from build123d import *

# Parameters (mm, degrees)
SKETCH1_R           = 1.5
SKETCH1_R_2         = 1.25
BOSS_EXTRUDE1_DEPTH = 3
SKETCH2_R           = 1.25
BOSS_EXTRUDE2_DEPTH = 3
SKETCH3_R           = 5
SKETCH3_R_2         = 3
BOSS_EXTRUDE3_DEPTH = 5
SKETCH3_2_R         = 3
SKETCH3_2_R_2       = 1.5
BOSS_EXTRUDE4_DEPTH = 1
CHAMFER1_SIZE       = 1.5


with BuildPart() as part:
    # Sketch1 → Boss-Extrude1 (new body)
    with BuildSketch(Plane(origin=(0, 0, 0), x_dir=(1, 0, 0), z_dir=(0, 1, 0))):
        with BuildLine():
            Line((-8.5, 6), (8.5, 6))
            ThreePointArc((8.5, 6), (14.5, 0), (8.5, -6))
            Line((8.5, -6), (-8.5, -6))
            ThreePointArc((-8.5, -6), (-14.5, 0), (-8.5, 6))
        make_face()
        with Locations((-8.5, 0)):
            Circle(SKETCH1_R, mode=Mode.SUBTRACT)
        with Locations((11.25, 0)):
            Circle(SKETCH1_R_2, mode=Mode.SUBTRACT)
        with Locations((6.25, 0)):
            Circle(SKETCH1_R_2, mode=Mode.SUBTRACT)
    extrude(amount=BOSS_EXTRUDE1_DEPTH)

    # Sketch2 → Boss-Extrude2 (add)
    with BuildSketch(Plane(origin=(0, 3, 0), x_dir=(1, 0, 0), z_dir=(0, 1, 0))):
        with BuildLine():
            Line((6, 3), (11.5, 3))
            ThreePointArc((11.5, 3), (14.5, 0), (11.5, -3))
            Line((11.5, -3), (6, -3))
            ThreePointArc((6, -3), (3, 0), (6, 3))
        make_face()
        with Locations((6.25, 0)):
            Circle(SKETCH2_R, mode=Mode.SUBTRACT)
        with Locations((11.25, 0)):
            Circle(SKETCH2_R, mode=Mode.SUBTRACT)
    extrude(amount=BOSS_EXTRUDE2_DEPTH)

    # Sketch3 → Boss-Extrude3 (add)
    with BuildSketch(Plane.XZ):
        with Locations((-8.5, 0)):
            Circle(SKETCH3_R)
        with Locations((-8.5, 0)):
            Circle(SKETCH3_R_2, mode=Mode.SUBTRACT)
    extrude(amount=BOSS_EXTRUDE3_DEPTH)

    # Sketch3<2> → Boss-Extrude4 (add)
    with BuildSketch(Plane.XZ):
        with Locations((-8.5, 0)):
            Circle(SKETCH3_2_R)
        with Locations((-8.5, 0)):
            Circle(SKETCH3_2_R_2, mode=Mode.SUBTRACT)
    extrude(amount=BOSS_EXTRUDE4_DEPTH)

    # Chamfer1
    chamfer1_edges = [part.edges().sort_by_distance(p)[0] for p in [
        (-10, 3, 0),
    ]]
    chamfer(chamfer1_edges, length=CHAMFER1_SIZE)


solid = part.part
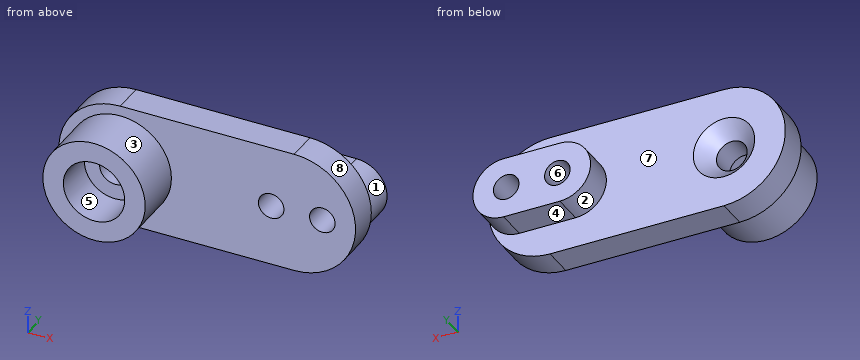
Work out the finished part from the listing and answer in its coordinate system (mm). Face numbers are marked on the shaded views. A direction names the side the tool comes from. Round coordinates to 2 decimals unless told otherwise and drop trailing zeros. Loops run counter-clockwise (first coordinate to the right, second up) from the corner with the lowest first, then second, coordinate; pieces in that order, holes last. Notation, with made-up numbers: (66, 9.5) - (113, 9.5) arc R14 ccw to (113, 31.5) - close; hole circle Ø2 at (23, -17.5). An arc over 180 degrees is marked (long way). Use one line per item in the form item = value. Start each with the question number.
(1) Determine the mould class of the marked faces 5, 6, 7 and 8 for opening direction X: +X half, -X half, draft (parallel to the pull), parting line (faces both ways), or undercut.
(2) Flat-ended cylindrical pins translate along their axes: P1, Ø2, axis at x = -4, z = 3, coming from the +Y side; P2, Ø3.5, axis at x = -8.5, z = 0, coming from the +Y side; P3, Ø0.9, axis at x = 8.5, y = 4, coming from the +Z side; P4, Ø1.5, axis at y = -0.5, z = -0.5, coming from the -X side. Find the tip coordinate at first contact, or state that the pin passes through.
(3) Find section D-D on y = -2.75. Determine the outline of the cut face in (x, z).
(4) Consider line 1 (X direction, y = 0.7, z = 0); line 2 (Y direction, x = -6.25, z = 5); line 3 (X direction, y = 3.5, z = -0.5). Determine where each line is inside the solid, lowest interval first.
(5) Find section C-C on z = -3.5. Determine the outline of the cut face in (x, y).
(6) Which of the six approach directions +Z, -Z, +X, -X, +Y, -Y give full straight-line access (tool end or side, diameter ignored) to the marked faces 1, 2, 3 and 4?
(7) Find section B-B on x = 4.5. Determine the outline of the cut face in (y, z), and give its area (3 significant figures).
(8) Find section A-A on y = 2.25. Determine the outline of the cut face in (x, z), and give its area (3 significant figures).
Answer list:
q1.face_5 = undercut
q1.face_6 = undercut
q1.face_7 = draft
q1.face_8 = +X half
q2.P1 = 3
q2.P2 = 1.75
q2.P3 = 3
q2.P4 = -14.5
q3.outline = circle Ø10 at (-8.5, 0); hole circle Ø6 at (-8.5, 0)
q4.line_1 = -14.5 to -10, -7 to 5, 7.5 to 10, 12.5 to 14.5
q4.line_2 = 0 to 3
q4.line_3 = 3.04 to 5.1, 7.4 to 10.1, 12.4 to 14.46
q5.outline = (-13.37, 0) - (-12.07, 0) - (-12.07, -5) - (-4.93, -5) - (-4.93, 0) - (13.37, 0) - (13.37, 3) - (-13.37, 3) - close
q6.face_1 = +X, +Y
q6.face_2 = -X, +Y
q6.face_3 = -Y
q6.face_4 = -Z, +X, -X, +Y
q7.outline = (0, -6) - (3, -6) - (3, -2.6) - (6, -2.6) - (6, 2.6) - (3, 2.6) - (3, 6) - (0, 6) - close
q7.area = 51.6 mm^2
q8.outline = (-8.5, -6) - (8.5, -6) arc R6 ccw to (8.5, 6) - (-8.5, 6) arc R6 ccw to start; hole circle Ø4.5 at (-8.5, 0); hole circle Ø2.5 at (6.25, 0); hole circle Ø2.5 at (11.25, 0)
q8.area = 291 mm^2
